```python
from build123d import *

# Parameters (mm, degrees)
SKETCH1_W                = 12.7
SKETCH1_H                = 6.5
BOSS_EXTRUDE1_DEPTH      = 5.75
SKETCH2_R                = 1.1
CUT_EXTRUDE1_DEPTH       = 6.75
SKETCH3_W                = 0.9
SKETCH3_H                = 3.5
BOSS_EXTRUDE2_DEPTH      = 0.2
BOSS_EXTRUDE2_DEPTH_BACK = 0.2
BOSS_EXTRUDE3_DEPTH      = 1.45
BOSS_EXTRUDE3_DEPTH_BACK = 1.45


with BuildPart() as part:
    # Sketch1 → Boss-Extrude1 (new body)
    with BuildSketch(Plane(origin=(0, 0, 0), x_dir=(1, 0, 0), z_dir=(0, 1, 0))):
        with Locations((6.35, 3.25)):
            Rectangle(SKETCH1_W, SKETCH1_H)
    extrude(amount=BOSS_EXTRUDE1_DEPTH)

    # Sketch2 → Cut-Extrude1 (cut, through all)
    with BuildSketch(Plane(origin=(0, 5.75, 0), x_dir=(1, 0, 0), z_dir=(0, 1, 0))):
        with Locations((3.1, 1.5)):
            Circle(SKETCH2_R)
        with Locations((9.6, 1.5)):
            Circle(SKETCH2_R)
    extrude(amount=-CUT_EXTRUDE1_DEPTH, mode=Mode.SUBTRACT)

    # Sketch3 → Boss-Extrude2 (add, two sides)
    with BuildSketch(Plane(origin=(0, 2.875, 0), x_dir=(1, 0, 0), z_dir=(0, 1, 0))) as boss_extrude2_sk:
        with Locations((6.35, -1.75)):
            Rectangle(SKETCH3_W, SKETCH3_H)
        Polygon((11.88, 0), (11.88, -3.5), (11.43, -3.5), (10.98, -3.5), (10.98, 0), align=None)
        Polygon((0.82, 0), (1.72, 0), (1.72, -3.5), (1.27, -3.5), (0.82, -3.5), align=None)
    extrude(amount=BOSS_EXTRUDE2_DEPTH)
    extrude(boss_extrude2_sk.sketch, amount=-BOSS_EXTRUDE2_DEPTH_BACK)

    # Sketch4 → Boss-Extrude3 (add, two sides)
    with BuildSketch(Plane(origin=(0, 2.875, 0), x_dir=(1, 0, 0), z_dir=(0, 1, 0))) as boss_extrude3_sk:
        with BuildLine():
            Line((3.8, 6.5), (5, 6.5))
            ThreePointArc((5, 6.5), (4.4, 7.1), (3.8, 6.5))
        make_face()
    extrude(amount=BOSS_EXTRUDE3_DEPTH)
    extrude(boss_extrude3_sk.sketch, amount=-BOSS_EXTRUDE3_DEPTH_BACK)


solid = part.part
```
Read the model definition and answer for the solid it produces. Units are mm, in the model's axes. A direction names the side the tool comes from. Coordinates: 2 decimals unless noted, no trailing zeros. Write each loop counter-clockwise with the first axis right and the second up, starting at its lowest first coordinate (ties: lowest second). Pieces come first, ordered by that corner, then holes. Notation, with made-up numbers: (-3, 68.25) -> (33, 68.25) arc R19 cw to (33, 74.25) -> close; hole circle Ø6 at (-0.5, 72.25). An arc over 180 degrees is marked (long way). Return JSON: item names as keys, results as strings.
1. A cutting plane is placed at B-B (x = 9.6). Determine the outline of the cut face in (y, z), and give its area (3 significant figures).
Found:
{"outline": "(0, -6.5) -> (5.75, -6.5) -> (5.75, -2.6) -> (0, -2.6) -> close; (0, -0.4) -> (5.75, -0.4) -> (5.75, 0) -> (0, 0) -> close", "area": "24.7 mm2"}
2. Each of these flat-tipped pins is pushed along its axis until it touches: P1, Ø1.5, axis at x = 8.5, y = 0.5, coming from the -Z side; P2, Ø0.7, axis at x = 11.5, z = 1.5, coming from the -Y side (3 decimals); P3, Ø1, axis at x = 9, z = -2, coming from the -Y side. Where does it stop, or does it pass through?
Found:
{"P1": "z = -6.5", "P2": "y = 2.675", "P3": "y = 0"}
3. A cutting plane is placed at C-C (y = 1.9). Determine the outline of the cut face in (x, z), and give its area (3 significant figures).
Found:
{"outline": "(0, -6.5) -> (3.8, -6.5) arc R0.6 ccw to (5, -6.5) -> (12.7, -6.5) -> (12.7, 0) -> (0, 0) -> close; hole circle Ø2.2 at (3.1, -1.5); hole circle Ø2.2 at (9.6, -1.5)", "area": "75.5 mm2"}
4. A tool of negligible diameter and unlimited length cuts with its end or side. For faces 4 (the face through (1, 2.675, 2)), 5 (the face through (1, 3.075, 2)), 6 (the face through (6, 5.75, -3)), from which of +Z, -Z, +X, -X, +Y, -Y can it reach the whole face along a straight path? Write none if from no direction.
Found:
{"face 4": "+Z, +X, -X, -Y", "face 5": "+Z, +X, -X, +Y", "face 6": "+Z, -Z, +X, -X, +Y"}
5. Determine the mould class of faces 1 (the face through (0, 3, -3)), 2 (the face through (4.4, 2.9, -7.1)), 3 (the face through (8.789, 2.915, -2.243)) for opening direction Z: pulls with the +Z half, pulls with the -Z half, needs draft (parallel to the pull), parting line crosses it, or undercut.
Found:
{"face 1": "needs draft", "face 2": "pulls with the -Z half", "face 3": "undercut"}
6. Find the intervals of material crossed by line 1 along X through (y, z) = (3.15, -1.5); line 2 along Z through (x, y) = (3.1, 2.8); line 3 along Z through (x, y) = (5.5, 4.4), in increasing order. Write a range as from..to.
Found:
{"line 1": "0..2, 4.2..8.5, 10.7..12.7", "line 2": "-6.5..-2.6, -0.4..0", "line 3": "-6.5..0"}
7. A cutting plane is placed at A-A (z = 2). Determine the outline of the cut face in (x, y) (3 decimals), and give its area (3 significant figures).
Found:
{"outline": "(0.82, 2.675) -> (1.72, 2.675) -> (1.72, 3.075) -> (0.82, 3.075) -> close; (5.9, 2.675) -> (6.8, 2.675) -> (6.8, 3.075) -> (5.9, 3.075) -> close; (10.98, 2.675) -> (11.88, 2.675) -> (11.88, 3.075) -> (10.98, 3.075) -> close", "area": "1.08 mm2"}
8. A cutting plane is placed at D-D (z = -1.5). Determine the outline of the cut face in (x, y).
Found:
{"outline": "(0, 0) -> (2, 0) -> (2, 5.75) -> (0, 5.75) -> close; (4.2, 0) -> (8.5, 0) -> (8.5, 5.75) -> (4.2, 5.75) -> close; (10.7, 0) -> (12.7, 0) -> (12.7, 5.75) -> (10.7, 5.75) -> close"}
